Could you check a few things on this model? Use its own coordinates, in mm. A direction names the side the tool comes from. Give positions to 0.01 mm unless a question says otherwise; leave off trailing zeros. Loops run counter-clockwise (first coordinate to the right, second up) from the corner with the lowest first, then second, coordinate; pieces in that order, holes last. Notation, with made-up numbers: (4.5, 40) - (28.5, 40) arc R18 ccw to (28.5, 73) - close; hole circle Ø4 at (-31.75, -22.75). An arc over 180 degrees is marked (long way). Use CSV: the item, a comma, the result in double quotes.
from build123d import *

# Parameters (mm, degrees)
SKETCH1_W          = 88.9
SKETCH1_H          = 4.7625
CHAMFER1_SIZE      = 1.190625
CUT_EXTRUDE2_DEPTH = 3.53822


with BuildPart() as part:
    # Sketch1 → Revolve1 (revolve)
    with BuildSketch(Plane(origin=(0, 0, 0), x_dir=(0, 0, -1), z_dir=(1, 0, 0))):
        with Locations((49.5046, 2.38125)):
            Rectangle(SKETCH1_W, SKETCH1_H)
    revolve(axis=Axis((0, 0, -93.9546), (0, 0, 1)))

    # Chamfer1
    chamfer1_edges = [part.edges().sort_by_distance(p)[0] for p in [
        (0, -4.7625, -93.9546),
    ]]
    chamfer(chamfer1_edges, length=CHAMFER1_SIZE)

    # Sketch7 → Revolve2 (revolve)
    with BuildSketch(Plane(origin=(0, 0, 0), x_dir=(0, 0, -1), z_dir=(1, 0, 0)), mode=Mode.PRIVATE) as revolve2_sk:
        with BuildLine():
            Line((4.29641, 8.3312), (5.0546, 8.3312))
            Line((5.0546, 8.3312), (5.0546, 0))
            Line((5.0546, 0), (0, 0))
            Line((0, 0), (0, 4.7625))
            ThreePointArc((0, 4.7625), (1.862939611, 6.890285164), (4.29641, 8.3312))
        make_face()
    revolve(revolve2_sk.sketch.rotate(Axis((0, 0, 0), (0, 0, -1)), 180), axis=Axis((0, 0, 0), (0, 0, -1)))

    # Sketch5 → Cut-Extrude2 (cut)
    with BuildSketch(Plane.XY):
        Polygon((2.778125, -1.603951217), (2.778125, 1.603951217), (0, 3.207902433), (-2.778125, 1.603951217), (-2.778125, -1.603951217), (0, -3.207902433), align=None)
    extrude(amount=-CUT_EXTRUDE2_DEPTH, mode=Mode.SUBTRACT)

    # Cut-Extrude3 cone 1 section (on through the dimple's axis) → Cut-Extrude3 (revolve, cut)
    with BuildSketch(Plane(origin=(0, 0, 0), x_dir=(0, -1, 0), z_dir=(1, 0, 0))):
        Polygon((0, 0), (3.207902433, 0), (0, 3.207902433), align=None)
    revolve(axis=Axis((0, 0, 0), (0, 0, -1)), mode=Mode.SUBTRACT)


solid = part.part
1) Which directions (+Z, -Z, +X, -X, +Y, -Y) give clear straight access to the entire face, cutting with the end or side of a thin tool? Please do faces 4 (the cylindrical face through (2.9, -3.78, -49.52)), 5 (the flat face through (-1.4, -2.4, -1.7)).
Answer below:
face 4,"-Z"
face 5,"+Z"
2) I need wall thicknesses on line 1 along Z through (x, y) = (-2.25, -0.5); line 2 along X through (y, z) = (-0.25, -83.5); line 3 along Z through (x, y) = (1, 7.5). Which ranges of each line are inside material? Lowest first, please.
Answer below:
line 1,"z = -93.95 to -3.54"
line 2,"x = -4.76 to 4.76"
line 3,"z = -5.05 to -2.79"
3) Suppose I cut it at C-C (x = -7.5). Please give me the cut outline in (y, z).
Answer below:
outline,"(-3.63, -5.05) - (3.63, -5.05) - (3.63, -4.3) arc R4.9 ccw to (-3.63, -4.3) - close"
4) Suppose I cut it at A-A (y = 0). Please give me the cut outline in (x, z), plus the area to 3 significant figures.
Answer below:
outline,"(-8.33, -5.05) - (-4.76, -5.05) - (-4.76, -92.76) - (-3.57, -93.95) - (3.57, -93.95) - (4.76, -92.76) - (4.76, -5.05) - (8.33, -5.05) - (8.33, -4.3) arc R8.96 ccw to (4.76, 0) - (3.21, 0) - (2.78, -0.43) - (2.78, -3.54) - (-2.78, -3.54) - (-2.78, -0.43) - (-3.21, 0) - (-4.76, 0) arc R8.96 ccw to (-8.33, -4.3) - close"
area,"898 mm2"
5) Suppose I cut it at D-D (y = -6.75). Please give me the cut outline in (x, z).
Answer below:
outline,"(-4.88, -5.05) - (4.88, -5.05) - (4.88, -4.3) arc R5.89 ccw to (-4.88, -4.3) - close"
6) Suppose I cut it at B-B (z = -19). Please give me the cut outline in (x, y) (1 decimal).
Answer below:
outline,"circle Ø9.5 at (0, 0)"
7) We'd pull the mould along Y, two halves only. Please class faces 1 (the conical face through (-1.476, -2.6, -0.218)), 2 (the cylindrical face through (-2.502, -7.946, -4.681)), 3 (the flat face through (0, 0, -93.955)): +Y half, -Y half, draft (parallel to the pull), parting line (faces both ways), or undercut.
Answer below:
face 1,"undercut"
face 2,"parting line"
face 3,"draft"
8) I'm going to push flat-ended pins straight in: P1, Ø5, axis at x = 5, z = -47, coming from the +Y side; P2, Ø8, axis at x = -0.5, z = -82, coming from the -Y side; P3, Ø4, axis at x = -6, y = -3.5, coming from the +Z side; P4, Ø6, axis at x = 1, y = -1, coming from the +Z side. Where does each tip first touch, or does it pass through?
Answer below:
P1,"stops at y = 4.05"
P2,"stops at y = -4.76"
P3,"stops at z = -0.12"
P4,"stops at z = 0"
